from build123d import *

# Parameters (mm, degrees)
CROQUIS1_W                                           = 12
CROQUIS1_H                                           = 250
SALIENTE_EXTRUIR1_DEPTH                              = 8
CORTAR_EXTRUIR1_DEPTH                                = 251.104793708
CORTAR_EXTRUIR2_DEPTH                                = 251.104793708
CORTAR_EXTRUIR3_DEPTH                                = 251.104793708
CORTAR_EXTRUIR4_DEPTH                                = 251.104793708
CORTAR_EXTRUIR5_DEPTH                                = 251.104793708
CORTAR_EXTRUIR6_DEPTH                                = 251.104793708
CORTAR_EXTRUIR7_DEPTH                                = 251.104793708
REFRENTADO_PARA_TORNILLO_CON_CABEZA_HEXA_D           = 3.5
REFRENTADO_PARA_TORNILLO_CON_CABEZA_HEXA_CBORE_D     = 6
REFRENTADO_PARA_TORNILLO_CON_CABEZA_HEXA_CBORE_DEPTH = 4.5
CHAFL_N1_SIZE                                        = 0.4
CHAFL_N2_SIZE                                        = 0.034056407
CHAFL_N2_SIZE_2                                      = 0.03688403
CHAFL_N3_SIZE                                        = 0.091173812
CHAFL_N3_SIZE_2                                      = 0.105000846


with BuildPart() as part:
    # Croquis1 → Saliente-Extruir1 (new body)
    with BuildSketch(Plane(origin=(0, 4.050658692, 0), x_dir=(1, 0, 0), z_dir=(0, 1, 0))):
        with Locations((0, 125)):
            Rectangle(CROQUIS1_W, CROQUIS1_H)
    extrude(amount=-SALIENTE_EXTRUIR1_DEPTH)

    # Croquis2 → Cortar-Extruir1 (cut, through all)
    with BuildSketch(Plane(origin=(0, 0, -250), x_dir=(-1, 0, 0), z_dir=(0, 0, -1))):
        with BuildLine():
            Line((1.35, -3.949341308), (1.85, -3.949341308))
            ThreePointArc((1.85, -3.949341308), (1.6, -3.849341308), (1.35, -3.949341308))
        make_face()
    extrude(amount=-CORTAR_EXTRUIR1_DEPTH, mode=Mode.SUBTRACT)

    # Croquis3 → Cortar-Extruir2 (cut, through all)
    with BuildSketch(Plane(origin=(0, 0, -250), x_dir=(-1, 0, 0), z_dir=(0, 0, -1))):
        with BuildLine():
            Line((-6, 2.100658692), (-6, 1.200658692))
            Line((-6, 1.200658692), (-5.2, 1.200658692))
            ThreePointArc((-5.2, 1.200658692), (-4.75, 1.650658692), (-5.2, 2.100658692))
            Line((-5.2, 2.100658692), (-6, 2.100658692))
        make_face()
    extrude(amount=-CORTAR_EXTRUIR2_DEPTH, mode=Mode.SUBTRACT)

    # Croquis4 → Cortar-Extruir3 (cut, through all)
    with BuildSketch(Plane(origin=(0, 0, -250), x_dir=(-1, 0, 0), z_dir=(0, 0, -1))):
        with BuildLine():
            Line((-5.622557264, 1.200658692), (-6, 1.200658692))
            Line((-6, 1.200658692), (-6, 0.689297919))
            ThreePointArc((-6, 0.689297919), (-5.684900038, 0.851696449), (-5.622557264, 1.200658692))
        make_face()
    extrude(amount=-CORTAR_EXTRUIR3_DEPTH, mode=Mode.SUBTRACT)

    # Croquis5 → Cortar-Extruir4 (cut, through all)
    with BuildSketch(Plane(origin=(0, 0, -250), x_dir=(-1, 0, 0), z_dir=(0, 0, -1))):
        with BuildLine():
            Line((-6, 2.612019466), (-6, 2.100658692))
            Line((-6, 2.100658692), (-5.622557264, 2.100658692))
            ThreePointArc((-5.622557264, 2.100658692), (-5.684900038, 2.449620935), (-6, 2.612019466))
        make_face()
    extrude(amount=-CORTAR_EXTRUIR4_DEPTH, mode=Mode.SUBTRACT)

    # Croquis6 → Cortar-Extruir5 (cut, through all)
    with BuildSketch(Plane(origin=(0, 0, -250), x_dir=(-1, 0, 0), z_dir=(0, 0, -1))):
        with BuildLine():
            Line((6, 1.200658692), (6, 2.100658692))
            Line((6, 2.100658692), (5.2, 2.100658692))
            ThreePointArc((5.2, 2.100658692), (4.75, 1.650658692), (5.2, 1.200658692))
            Line((5.2, 1.200658692), (6, 1.200658692))
        make_face()
    extrude(amount=-CORTAR_EXTRUIR5_DEPTH, mode=Mode.SUBTRACT)

    # Croquis7 → Cortar-Extruir6 (cut, through all)
    with BuildSketch(Plane(origin=(0, 0, -250), x_dir=(-1, 0, 0), z_dir=(0, 0, -1))):
        with BuildLine():
            Line((5.622557264, 2.100658692), (6, 2.100658692))
            Line((6, 2.100658692), (6, 2.612019466))
            ThreePointArc((6, 2.612019466), (5.684900038, 2.449620935), (5.622557264, 2.100658692))
        make_face()
    extrude(amount=-CORTAR_EXTRUIR6_DEPTH, mode=Mode.SUBTRACT)

    # Croquis8 → Cortar-Extruir7 (cut, through all)
    with BuildSketch(Plane(origin=(0, 0, -250), x_dir=(-1, 0, 0), z_dir=(0, 0, -1))):
        with BuildLine():
            Line((6, 0.689297919), (6, 1.200658692))
            Line((6, 1.200658692), (5.622557264, 1.200658692))
            ThreePointArc((5.622557264, 1.200658692), (5.684900038, 0.851696449), (6, 0.689297919))
        make_face()
    extrude(amount=-CORTAR_EXTRUIR7_DEPTH, mode=Mode.SUBTRACT)

    # Refrentado para tornillo con cabeza hexagonal de M31 (through all)
    with Locations(Plane(origin=(0, 4.050658692, 0), x_dir=(1, 0, 0), z_dir=(0, 1, 0))):
        with Locations((0, 45), (0, 65), (0, 85), (0, 105), (0, 125), (0, 145), (0, 165), (0, 185), (0, 205), (0, 225), (0, 245), (0, 25), (-0.275406539, 5)):
            CounterBoreHole(REFRENTADO_PARA_TORNILLO_CON_CABEZA_HEXA_D / 2, REFRENTADO_PARA_TORNILLO_CON_CABEZA_HEXA_CBORE_D / 2, REFRENTADO_PARA_TORNILLO_CON_CABEZA_HEXA_CBORE_DEPTH)

    # Chaflán1
    chafl_n1_edges = [part.edges().sort_by_distance(p)[0] for p in [
        (-6, -3.949341308, -125),
        (6, -3.949341308, -125),
        (-6, 4.050658692, -125),
        (6, 4.050658692, -125),
    ]]
    chamfer(chafl_n1_edges, length=CHAFL_N1_SIZE)

    # Chaflán2
    # the kernel refuses this chamfer: 0.03688403, 0.034056407 mm, written as the material it takes off along each edge
    with BuildSketch(Plane(origin=(6, 0.689297919, -250.100435582), x_dir=(-0.9978479381588691, 0.06557051404475742, 0), z_dir=(0, 0, 1))) as chafl_n2_piece_1:
        with BuildLine():
            Line((0.03902449, 0), (-CHAFL_N2_SIZE * 0.0655705141026, CHAFL_N2_SIZE * 0.997847939043))
            Line((-CHAFL_N2_SIZE * 0.0655705141026, CHAFL_N2_SIZE * 0.997847939043), (0, 0))
            ThreePointArc((0, 0), (0.020082989, 0.000475786), (0.03902449, 0))
        make_face()
    extrude(amount=250.200871164, mode=Mode.SUBTRACT)
    with BuildSketch(Plane(origin=(6, 2.612019466, -250.094971685), x_dir=(0, 1, 0), z_dir=(0, 0, 1))) as chafl_n2_piece_2:
        with BuildLine():
            Line((CHAFL_N2_SIZE_2 * 0.999999990825, 0), (-0.002179894, 0.035512658))
            ThreePointArc((-0.002179894, 0.035512658), (-0.000727719, 0.018309495), (0, 0))
            Line((0, 0), (CHAFL_N2_SIZE_2 * 0.999999990825, 0))
        make_face()
    extrude(amount=250.189943371, mode=Mode.SUBTRACT)
    with BuildSketch(Plane(origin=(-6, 2.612019466, -250.100435582), x_dir=(0, 1, 0), z_dir=(0, 0, 1))) as chafl_n2_piece_3:
        with BuildLine():
            Line((CHAFL_N2_SIZE, 0), (-0.002558856, -0.038940507))
            ThreePointArc((-0.002558856, -0.038940507), (-0.00084209, -0.020070966), (0, 0))
            Line((0, 0), (CHAFL_N2_SIZE, 0))
        make_face()
    extrude(amount=250.200871164, mode=Mode.SUBTRACT)
    with BuildSketch(Plane(origin=(-6, 0.689297919, -250.094971685), x_dir=(0.9981213351064977, 0.061268265890444186, 0), z_dir=(0, 0, 1))) as chafl_n2_piece_4:
        with BuildLine():
            Line((0.0355795, 0), (-CHAFL_N2_SIZE_2 * 0.0612682653277, -CHAFL_N2_SIZE_2 * 0.998121325949))
            Line((-CHAFL_N2_SIZE_2 * 0.0612682653277, -CHAFL_N2_SIZE_2 * 0.998121325949), (0, 0))
            ThreePointArc((0, 0), (0.018319684, -0.000395439), (0.0355795, 0))
        make_face()
    extrude(amount=250.189943371, mode=Mode.SUBTRACT)

    # Chaflán3
    # the kernel refuses this chamfer: 0.105000846, 0.091173812 mm, written as the material it takes off along each edge
    with BuildSketch(Plane(origin=(5.622557264, 1.200658692, -250.318147751), x_dir=(-0.1263625484615496, -0.991984126055605, 0), z_dir=(0, 0, 1)), Plane(origin=(-5.622557264, 2.100658692, -250.318147751), x_dir=(0.12636254846156672, 0.9919841260556028, 0), z_dir=(0, 0, 1))) as chafl_n3_piece_1:
        with BuildLine():
            Line((0.123959197, 0), (CHAFL_N3_SIZE * 0.126362548546, -CHAFL_N3_SIZE * 0.99198412672))
            Line((CHAFL_N3_SIZE * 0.126362548546, -CHAFL_N3_SIZE * 0.99198412672), (0, 0))
            ThreePointArc((0, 0), (0.063641461, -0.004827559), (0.123959197, 0))
        make_face()
    extrude(amount=250.636295502, mode=Mode.SUBTRACT)
    with BuildSketch(Plane(origin=(5.622557264, 2.100658692, -250.269677179), x_dir=(-1, 0, 0), z_dir=(0, 0, 1)), Plane(origin=(-5.622557264, 1.200658692, -250.269677179), x_dir=(1, 0, 0), z_dir=(0, 0, 1))) as chafl_n3_piece_2:
        with BuildLine():
            Line((CHAFL_N3_SIZE_2, 0), (0.015616157, -0.098323158))
            ThreePointArc((0.015616157, -0.098323158), (0.011085216, -0.04998658), (0, 0))
            Line((0, 0), (CHAFL_N3_SIZE_2, 0))
        make_face()
    extrude(amount=250.539354358, mode=Mode.SUBTRACT)


solid = part.part
Here's how the part is built. I have some questions about the finished solid (model axes, mm). A direction names the side the tool comes from. Give positions to 0.01 mm unless a question says otherwise; leave off trailing zeros. Use one line per item in the form item = value. Start each with the question number.
1. On a 3-axis mill with a long thin cutter (end or side, diameter ignored), from which of +Z, -Z, +X, -X, +Y, -Y can I reach the whole of each face in a straight line? I mean faces 5 (the face through (2, -0.449, -105)), 6 (the face through (0, 0, 0)). Say none if no direction works.
2. If I drill on L1, parallel to Y at x = 5.25, z = -95; L2, parallel to X at y = -1.3, z = -245; L3, parallel to X at y = 0.65, z = -245, over which ranges is the centre line in solid material (lowest first)?
3. Thinking about a two-plate mould opening in X: for faces 1 (the face through (0, 2, -208)), 2 (the face through (6, -1, -123)), 3 (the face through (0, 2, -48)), 4 (the face through (-3, 4.051, -127)), which applies, +X half, -X half, draft (parallel to the pull), parting line (faces both ways), or undercut?
4. Will this pin go through, and if not, where does the flat tip stop? pin 1 Ø1.8 at (x, z) = (0.5, -84) entering from +Y.
Entries:
q1.face_5 = +Y
q1.face_6 = +Z, +X, -X, +Y, -Y
q2.L1 = -3.95 to 1.2, 2.1 to 4.05
q2.L2 = -6 to -1.75, 1.75 to 6
q2.L3 = -6 to -3, 3 to 6
q3.face_1 = undercut
q3.face_2 = +X half
q3.face_3 = undercut
q3.face_4 = draft
q4.pin_1 = -0.45
